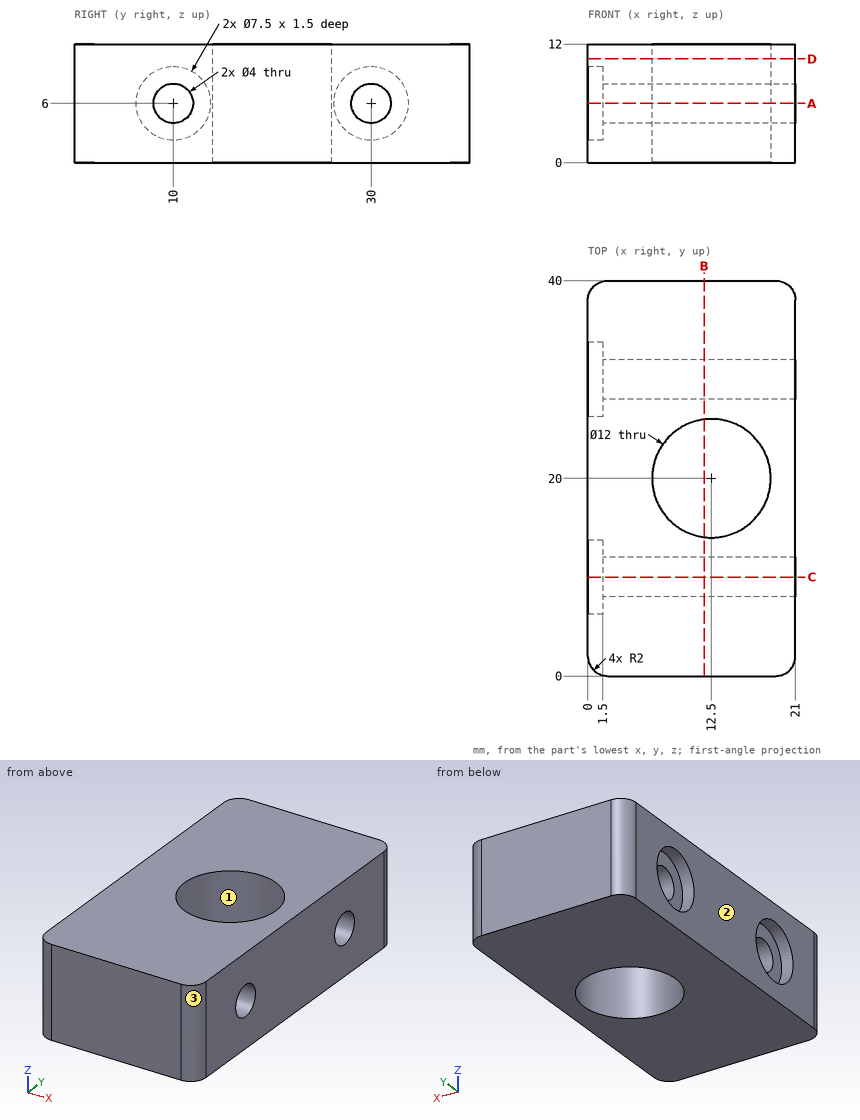
Study the drawing (mm; zero at the part's minimum x, y, z) and answer. Round coordinates to 2 decimals unless told otherwise and drop trailing zeros. Write each loop counter-clockwise with the first axis right and the second up, starting at its lowest first coordinate (ties: lowest second). Pieces come first, ordered by that corner, then holes. Notation, with made-up numbers: (-25, 6.25) - (-3, 6.25) arc R6 cw to (-3, 11.25) - close; hole circle Ø2 at (-33.75, 39). An arc over 180 degrees is marked (long way). Use CSV: the item, a comma, the result in double quotes.
Q1. Find section D-D, the plane z = 10.5. Write down the section's boundary in (x, y), then the cut area to 3 significant figures.
Values:
outline,"(0, 2) arc R2 ccw to (2, 0) - (19, 0) arc R2 ccw to (21, 2) - (21, 38) arc R2 ccw to (19, 40) - (2, 40) arc R2 ccw to (0, 38) - close; hole circle Ø12 at (12.5, 20)"
area,"723 mm²"
Q2. Find section A-A, the plane z = 6. Write down the section's boundary in (x, y), then the cut area to 3 significant figures.
Values:
outline,"(0, 2) arc R2 ccw to (2, 0) - (19, 0) arc R2 ccw to (21, 2) - (21, 8) - (1.5, 8) - (1.5, 6.25) - (0, 6.25) - close; (0, 13.75) - (1.5, 13.75) - (1.5, 12) - (21, 12) - (21, 28) - (1.5, 28) - (1.5, 26.25) - (0, 26.25) - close; (0, 33.75) - (1.5, 33.75) - (1.5, 32) - (21, 32) - (21, 38) arc R2 ccw to (19, 40) - (2, 40) arc R2 ccw to (0, 38) - close; hole circle Ø12 at (12.5, 20)"
area,"545 mm²"
Q3. Find section B-B, the plane x = 11.75. Write down the section's boundary in (y, z), then the cut area to 3 significant figures.
Values:
outline,"(0, 0) - (14.05, 0) - (14.05, 12) - (0, 12) - close; (25.95, 0) - (40, 0) - (40, 12) - (25.95, 12) - close; hole circle Ø4 at (10, 6); hole circle Ø4 at (30, 6)"
area,"312 mm²"
Q4. Find section C-C, the plane y = 10. Write down the section's boundary in (x, z), then the cut area to 3 significant figures.
Values:
outline,"(0, 0) - (21, 0) - (21, 4) - (1.5, 4) - (1.5, 2.25) - (0, 2.25) - close; (0, 9.75) - (1.5, 9.75) - (1.5, 8) - (21, 8) - (21, 12) - (0, 12) - close"
area,"163 mm²"
Q5. Straight lines are drawn through the part: line 1 along Y through (x, z) = (12, 5); line 2 along Y through (x, z) = (6, 6); line 3 along Y through (x, z) = (3.25, 7.5). For each, find the intervals that lie inside material, in ascending order.
Values:
line 1,"y = 0 to 8.27, 11.73 to 14.02, 25.98 to 28.27, 31.73 to 40"
line 2,"y = 0 to 8, 12 to 28, 32 to 40"
line 3,"y = 0 to 8.68, 11.32 to 28.68, 31.32 to 40"
Q6. Determine the mould class of the marked faces 1, 2 and 3 for opening direction Y: +Y half, -Y half, draft (parallel to the pull), parting line (faces both ways), or undercut.
Values:
face 1,"undercut"
face 2,"draft"
face 3,"-Y half"
Q7. Each of these flat-tipped pins is pushed along its axis until it touches: pin 1 Ø6.5 at (y, z) = (30, 6) entering from +X; pin 2 Ø2 at (y, z) = (31, 7) entering from -X; pin 3 Ø11 at (x, y) = (12.5, 20) entering from -Z. Where does it stop, or does it pass through?
Values:
pin 1,"stops at x = 21"
pin 2,"stops at x = 1.5"
pin 3,"passes through"
